The model under review builds one solid part; all positions refer to its coordinate system, in mm. A direction names the side the tool comes from. Give positions to 0.01 mm unless a question says otherwise; leave off trailing zeros. Order: outer loops, then holes, each group sorted by start corner. A loop starts at its lowest first (then second) coordinate and runs counter-clockwise, first axis right, second up. Notation, with made-up numbers: (20, 45) - (35, 45) arc R25 ccw to (35, 71) - close; hole circle Ø7 at (12, -27.75). An arc over 180 degrees is marked (long way). Put each result on its own line as item: value.
```python
from build123d import *

# Parameters (mm, degrees)
F0_W          = 300
F0_H          = 300
F1_DEPTH      = 20
F2_R          = 50
F3_DEPTH      = 200
F3_DEPTH_BACK = 200
F5_R          = 50
F6_DEPTH      = 200
F6_DEPTH_BACK = 35


with BuildPart() as f1:
    # F0 (on Front) → F1 (new body)
    with BuildSketch(Plane.XZ):
        with Locations((7.894735, 0)):
            Rectangle(F0_W, F0_H)
    extrude(amount=F1_DEPTH)

    # F2 (on face) → F3 (join, two sides)
    with BuildSketch(Plane.XZ.offset(20)) as f3_sk:
        with Locations((-80.105265, 88)):
            Circle(F2_R)
    extrude(amount=F3_DEPTH)
    extrude(f3_sk.sketch, amount=-F3_DEPTH_BACK)

    # F5 (on face) → F6 (join, two sides)
    with BuildSketch(Plane(origin=(0, -75, 75), x_dir=(1, 0, 0), z_dir=(0, -0.707107, 0.707107))) as f6_sk:
        Circle(F5_R)
    extrude(amount=F6_DEPTH)
    extrude(f6_sk.sketch, amount=-F6_DEPTH_BACK)


solid = f1.part
```
(1) Take a section at A-A, the plane y = 123. Write out the cut boundary in (x, z).
The answers:
outline: circle Ø100 at (-80.11, 88)
(2) Wall thickness on L1, parallel to Y at x = 66, z = 148.5; L2, parallel to Y at x = 27.5, z = 92; L3, parallel to Z at x = -64.5, y = -143: over which ranges is each line inside the solid? List them lowest first.
The answers:
L1: -20 to 0
L2: -151.06 to -32.94, -20 to 0
L3: 40.5 to 135.5
(3) Clearance check with flat-ended pins moving along their axes: pin 1 Ø16 at (x, y) = (46.5, -11) entering from +Z; pin 2 Ø4 at (x, y) = (-1, -186.5) entering from +Z; pin 3 Ø1.5 at (x, z) = (32.5, 32.5) entering from -Y. State where each tip first meets the part, or that it passes through.
The answers:
pin 1: z = 150
pin 2: z = 248.34
pin 3: y = -87.4
(4) The part is to be moulded in two halves that separate along Y. For faces 6 (the flat face through (-0.7, -52.3, 48.2)), 7 (the flat face through (6, -10, -150)), 8 (the flat face through (6, 0, 2)), say which applies: pulls with the +Y half, pulls with the -Y half, needs draft (parallel to the pull), parting line crosses it, or undercut.
The answers:
face 6: undercut
face 7: needs draft
face 8: pulls with the +Y half
(5) For faces 1 (the flat face through (-81, 180, 89)), 2 (the flat face through (-81, -220, 89)), 3 (the cylindrical face through (-119.8, 88.7, 57.6)), 4 (the flat face through (6, -10, 150)), 5 (the flat face through (-0.7, -215.926, 216.916)), list the 3-axis set-ups (+Z, -Z, +X, -X, +Y, -Y) from which the entire face can be reached by the end or side of a thin tool; tool diameter is ignored.
The answers:
face 1: +Z, -Z, +X, -X, +Y
face 2: -Z, +X, -X, -Y
face 3: +Y
face 4: +Z, +X, -X, +Y
face 5: +Z, +X, -X, -Y
(6) Take a section at D-D, the plane x = -117. Write out the cut boundary in (y, z), then the cut area to 3 significant figures.
The answers:
outline: (-220, 54.25) - (-20, 54.25) - (-20, -150) - (0, -150) - (0, 54.25) - (180, 54.25) - (180, 121.75) - (0, 121.75) - (0, 150) - (-20, 150) - (-20, 121.75) - (-220, 121.75) - close
area: 31,600 mm^2
(7) Take a section at B-B, the plane z = 8. Write out the cut boundary in (x, y).
The answers:
outline: (-142.11, -20) - (157.89, -20) - (157.89, 0) - (-142.11, 0) - close
(8) Take a section at C-C, the plane x = 68. Write out the cut boundary in (y, z), then the cut area to 3 significant figures.
The answers:
outline: (-20, -150) - (0, -150) - (0, 150) - (-20, 150) - close
area: 6,000 mm^2
